```python
from build123d import *

# Parameters (mm, degrees)
FILLET1_R          = 3
SKETCH3_R          = 5
CUT_EXTRUDE1_DEPTH = 322.947200755


with BuildPart() as part:
    # Sketch2 → Revolve1 (revolve)
    with BuildSketch(Plane(origin=(0, 0, 0), x_dir=(1, 0, 0), z_dir=(0, 1, 0))):
        Polygon((-160, 0), (160, 0), (160, -25), (140, -25), (140, -15), (-140, -15), (-140, -25), (-160, -25), align=None)
    revolve(axis=Axis((-179.615783414, 0, 0), (1, 0, 0)))

    # Fillet1
    fillet1_edges = [part.edges().sort_by_distance(p)[0] for p in [
        (140, 0, -25),
        (160, 0, -25),
        (-160, 0, -25),
        (-140, 0, -25),
    ]]
    fillet(fillet1_edges, radius=FILLET1_R)

    # Sketch3 → Cut-Extrude1 (cut, through all)
    with BuildSketch(Plane(origin=(160, 0, 0), x_dir=(0, 0, -1), z_dir=(1, 0, 0))):
        Circle(SKETCH3_R)
    extrude(amount=-CUT_EXTRUDE1_DEPTH, mode=Mode.SUBTRACT)


solid = part.part
```
Design review of the part built by this model. Coordinates are the model's own, in mm. A direction names the side the tool comes from. Coordinates: 2 decimals unless noted, no trailing zeros. Order: outer loops, then holes, each group sorted by start corner. A loop starts at its lowest first (then second) coordinate and runs counter-clockwise, first axis right, second up. Notation, with made-up numbers: (26.25, 72.25) -> (71.25, 72.25) arc R25 cw to (71.25, 91.25) -> close; hole circle Ø4 at (40, -16.75). An arc over 180 degrees is marked (long way). One line per item, written item: value. Start each with the question number.
Q1. For probe 1 along X at (y, z) = (-17, 6); probe 2 along Y at (x, z) = (57, 0); probe 3 along Z at (x, y) = (-116.5, 1), list the stretches that pass through material, from the lowest coordinate up.
Q2. Insertion check: pin 1 Ø12 at (x, y) = (-6.5, 2.5) entering from +Z; pin 2 Ø1 at (x, z) = (49.5, 8) entering from +Y; pin 3 Ø12 at (x, y) = (11.5, -10.5) entering from -Z; pin 4 Ø6 at (y, z) = (0, 0) entering from +X. Each pin has a flat end and moves straight along its axis. Give the tip position at first contact, or say it passes through.
Q3. Mouldability with a two-part tool opening along Z and no side actions: class faces 1 (the flat face through (-160, -5.2, -0.3)), 2 (the cylindrical face through (-150.098, -7.509, 23.846)), 3 (the cylindrical face through (2.24, -4.88, 1.08)) as pulls with the +Z half, pulls with the -Z half, needs draft (parallel to the pull), parting line crosses it, or undercut.
Q4. Take a section at A-A, the plane z = 0. State the section outline as (x, y) points.
Q5. Take a section at C-C, the plane x = 127.5. State the section outline as (y, z) points.
Q6. Tool access review of faces 4 (the flat face through (160, -5.2, 0.3)), 5 (the flat face through (-140, -5.2, -14.4)): name each direction out of +Z, -Z, +X, -X, +Y, -Y from which nothing blocks a thin tool from reaching the whole face with its end or side.
Values follow:
1. probe 1: x = -160 to -140, 140 to 160
1. probe 2: y = -15 to -5, 5 to 15
1. probe 3: z = -14.97 to -4.9, 4.9 to 14.97
2. pin 1: stops at z = 15
2. pin 2: stops at y = 12.99
2. pin 3: stops at z = -14.31
2. pin 4: passes through
3. face 1: needs draft
3. face 2: parting line crosses it
3. face 3: undercut
4. outline: (-160, -22) arc R3 ccw to (-157, -25) -> (-143, -25) arc R3 ccw to (-140, -22) -> (-140, -15) -> (140, -15) -> (140, -22) arc R3 ccw to (143, -25) -> (157, -25) arc R3 ccw to (160, -22) -> (160, -5) -> (-160, -5) -> close; (-160, 5) -> (160, 5) -> (160, 22) arc R3 ccw to (157, 25) -> (143, 25) arc R3 ccw to (140, 22) -> (140, 15) -> (-140, 15) -> (-140, 22) arc R3 ccw to (-143, 25) -> (-157, 25) arc R3 ccw to (-160, 22) -> close
5. outline: circle Ø30 at (0, 0); hole circle Ø10 at (0, 0)
6. face 4: +Z, -Z, +X, +Y, -Y
6. face 5: none
